Check sheet for the modelled part. Datum: model origin and axes. Units: mm. Face numbers are marked on the shaded views. A direction names the side the tool comes from. Give positions to 0.01 mm unless a question says otherwise; leave off trailing zeros. Write each loop counter-clockwise with the first axis right and the second up, starting at its lowest first coordinate (ties: lowest second). Pieces come first, ordered by that corner, then holes. Notation, with made-up numbers: (-12.75, -33.5) -> (3.25, -33.5) arc R18 cw to (3.25, -23.5) -> close; hole circle Ø7 at (48, -23). An arc over 180 degrees is marked (long way). Use a Markdown table: item, result. Add a question column.
1. Scan lines: probe 1 along Y at (x, z) = (311.5, -354.5); probe 2 along Y at (x, z) = (-470.5, 923); probe 3 along X at (y, z) = (614, -510). Record each from-to range of solid material in increasing order. Write a range as [from, to].
2. Cross-section at C-C (x = 473). Enter the section's corners in (y, z), then the cut area to 3 significant figures.
3. Cross-section at D-D (z = 122). Enter the section's corners in (x, y), then the cut area to 3 significant figures.
4. Cross-section at A-A (y = 1205). Enter the section's corners in (x, z), then the cut area to 3 significant figures.
5. Gauge pin test, flat ends, axial feed: P1, Ø1.5, axis at x = 118.5, y = 587.5, coming from the +Z side; P2, Ø2.5, axis at x = 608, z = 483.5, coming from the -Y side; P3, Ø5, axis at y = 1253, z = -138, coming from the -X side. Record the tip position at first contact, or that the pin passes through.
6. Release check for a two-part mould opening along Y. For the marked faces 3, 4, 5 and 6 record: released by +Y, released by -Y, zero draft, split by the parting line, or undercut.
7. Set-up check for the marked faces 1 and 2: record each of +Z, -Z, +X, -X, +Y, -Y from which the full face is reachable in a straight line by a thin tool's end or side.
8. Cross-section at B-B (z = -274). Enter the section's corners in (x, y).
from build123d import *

# Parameters (mm, degrees)
F0_R      = 76.2
F1_DEPTH  = 203.2
F1_FACE_R = 76.2
F2_DEPTH  = 25.4
F5_DEPTH  = 609.6
F6_R      = 254
F7_DEPTH  = 1488.44


with BuildPart() as f1:
    # F0 (on Front) → F1 (new body)
    with BuildSketch(Plane.XZ):
        with BuildLine():
            Line((606.582717, -823.478018), (606.582717, 1056.121982))
            Line((606.582717, 1056.121982), (-409.417283, 1056.121982))
            ThreePointArc((-409.417283, 1056.121982), (-553.101381, 996.60608), (-612.617283, 852.921982))
            Line((-612.617283, 852.921982), (-612.617283, -620.278018))
            ThreePointArc((-612.617283, -620.278018), (-553.101381, -763.962116), (-409.417283, -823.478018))
            Line((-409.417283, -823.478018), (606.582717, -823.478018))
        make_face()
        with Locations((-409.417283, -620.278018)):
            Circle(F0_R, mode=Mode.SUBTRACT)
        with Locations((-409.417283, 852.921982)):
            Circle(F0_R, mode=Mode.SUBTRACT)
    extrude(amount=F1_DEPTH)

    # F1_face (on face) → F2 (join)
    with BuildSketch(Plane(origin=(8.078428, 0, 116.321982), x_dir=(1, 0, 0), z_dir=(0, 1, 0))):
        with BuildLine():
            Line((598.504289, -939.8), (598.504289, 939.8))
            Line((598.504289, 939.8), (-417.495711, 939.8))
            ThreePointArc((-417.495711, 939.8), (-561.179808, 880.284098), (-620.695711, 736.6))
            Line((-620.695711, 736.6), (-620.695711, -736.6))
            ThreePointArc((-620.695711, -736.6), (-561.179808, -880.284098), (-417.495711, -939.8))
            Line((-417.495711, -939.8), (598.504289, -939.8))
        make_face()
        with Locations((-417.495711, 736.6)):
            Circle(F1_FACE_R, mode=Mode.SUBTRACT)
        with Locations((-417.495711, -736.6)):
            Circle(F1_FACE_R, mode=Mode.SUBTRACT)
    extrude(amount=F2_DEPTH)

    # F4 (on Right) → F5 (join)
    with BuildSketch(Plane.YZ):
        with BuildLine():
            Line((25.4, -823.478018), (1016, -823.478018))
            ThreePointArc((1016, -823.478018), (1445.829228, -522.094174), (1308.976107, -15.283943))
            Line((1308.976107, -15.283943), (25.4, 1056.121982))
            Line((25.4, 1056.121982), (25.4, -823.478018))
        make_face()
    extrude(amount=F5_DEPTH)

    # F6 (on face) → F7 (cut)
    with BuildSketch(Plane.YZ):
        with Locations((1016, -366.278018)):
            Circle(F6_R)
    extrude(amount=F7_DEPTH, mode=Mode.SUBTRACT)


solid = f1.part
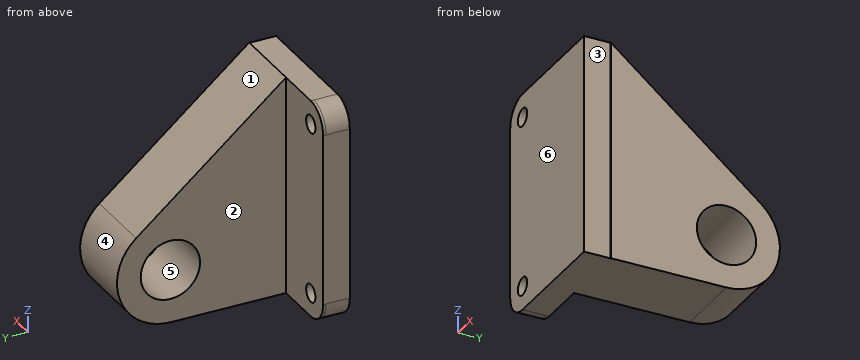
Worked answers:
| question | item | result |
|---|---|---|
| 1 | probe 1 | y = [-203.2, 762.27], [1269.73, 1473.05] |
| 1 | probe 2 | y = [-203.2, 25.4] |
| 1 | probe 3 | x = [0, 609.6] |
| 2 | outline | (-203.2, -823.48) -> (1016, -823.48) arc R457.2 ccw to (1308.98, -15.28) -> (25.4, 1056.12) -> (-203.2, 1056.12) -> close; hole circle Ø508 at (1016, -366.28) |
| 2 | area | 2,020,000 mm² |
| 3 | outline | (-612.62, -203.2) -> (606.58, -203.2) -> (606.58, 25.4) -> (609.6, 25.4) -> (609.6, 1144.51) -> (0, 1144.51) -> (0, 25.4) -> (-612.62, 25.4) -> close |
| 3 | area | 961,000 mm² |
| 4 | outline | (0, -782.58) -> (609.6, -782.58) -> (609.6, -535.97) -> (0, -535.97) -> close; (0, -196.59) -> (609.6, -196.59) -> (609.6, 71.51) -> (0, 71.51) -> close |
| 4 | area | 314,000 mm² |
| 5 | P1 | stops at z = 587.56 |
| 5 | P2 | stops at y = 25.4 |
| 5 | P3 | stops at x = 0 |
| 6 | face 3 | zero draft |
| 6 | face 4 | released by +Y |
| 6 | face 5 | undercut |
| 6 | face 6 | released by -Y |
| 7 | face 1 | +Z, +X, -X, +Y |
| 7 | face 2 | +Z, -Z, -X, +Y |
| 8 | outline | (-612.62, -203.2) -> (606.58, -203.2) -> (606.58, 25.4) -> (609.6, 25.4) -> (609.6, 779.36) -> (0, 779.36) -> (0, 25.4) -> (-612.62, 25.4) -> close; (0, 1252.64) -> (609.6, 1252.64) -> (609.6, 1463.79) -> (0, 1463.79) -> close |
